Model file for the job. Use its own axes, mm. Coordinates: 2 decimals unless noted, no trailing zeros. Write each loop counter-clockwise with the first axis right and the second up, starting at its lowest first coordinate (ties: lowest second). Pieces come first, ordered by that corner, then holes. Notation, with made-up numbers: (70, 70) -> (92, 70) arc R27 cw to (92, 93) -> close; hole circle Ø3 at (-31, 69). An arc over 180 degrees is marked (long way). Answer as a JSON object with one key per item and string values. Group by question number.
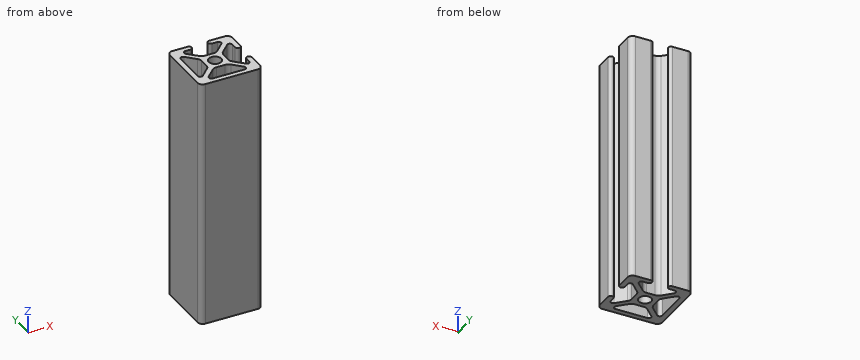
Autodesk Inventor part; units mm, degrees
ref_plane "YZ Plane" through (0, 0, 0) normal (1, 0, 0) x (0, 1, 0)
ref_plane "XZ Plane" through (0, 0, 0) normal (0, 1, 0) x (-1, 0, 0)
ref_plane "XY Plane" through (0, 0, 0) normal (0, 0, 1) x (1, 0, 0)
sketch "Sketch1" plane through (0, 0, 0) normal (0, 0, 1) x (1, 0, 0)
  arc A0 (-10.36, -6.4282) -> (-8.6498, -7.1366) centre (-9.3582, -6.4282) ccw
  line L0 (-10.36, 6.4282) -> (-10.36, -6.4282)
  arc A1 (-8.6498, 7.1366) -> (-10.36, 6.4282) centre (-9.3582, 6.4282) ccw
  line L1 (-5.1567, 3.6435) -> (-8.6498, 7.1366)
  arc A2 (-4.38, 1.7684) -> (-5.1567, 3.6435) centre (-7.0317, 1.7684) ccw
  line L2 (-4.38, -1.7684) -> (-4.38, 1.7684)
  arc A3 (-5.1567, -3.6435) -> (-4.38, -1.7684) centre (-7.0317, -1.7684) ccw
  line L3 (-8.6498, -7.1366) -> (-5.1567, -3.6435)
  arc A4 (-1.7684, -4.38) -> (-3.6435, -5.1567) centre (-1.7684, -7.0317) ccw
  line L4 (1.7684, -4.38) -> (-1.7684, -4.38)
  arc A5 (3.6435, -5.1567) -> (1.7684, -4.38) centre (1.7684, -7.0317) ccw
  line L5 (7.1366, -8.6498) -> (3.6435, -5.1567)
  arc A6 (6.4282, -10.36) -> (7.1366, -8.6498) centre (6.4282, -9.3582) ccw
  line L6 (-6.4282, -10.36) -> (6.4282, -10.36)
  arc A7 (-7.1366, -8.6498) -> (-6.4282, -10.36) centre (-6.4282, -9.3582) ccw
  line L7 (-3.6435, -5.1567) -> (-7.1366, -8.6498)
  circle A8 centre (0, 0) radius 2.5
  arc A9 (-4.32, 10.36) -> (-4.32, 12.5) centre (-4.32, 11.43) ccw
  line L8 (-4.32, 12.5) -> (-10.5183, 12.5)
  arc A10 (-10.5183, 12.5) -> (-12.5, 10.5183) centre (-10.5183, 10.5183) ccw
  line L9 (-12.5, 10.5183) -> (-12.5, -10.5183)
  arc A11 (-12.5, -10.5183) -> (-10.5183, -12.5) centre (-10.5183, -10.5183) ccw
  line L10 (-10.5183, -12.5) -> (10.5183, -12.5)
  arc A12 (10.5183, -12.5) -> (12.5, -10.5183) centre (10.5183, -10.5183) ccw
  line L11 (12.5, -10.5183) -> (12.5, -4.32)
  arc A13 (12.5, -4.32) -> (10.36, -4.32) centre (11.43, -4.32) ccw
  line L12 (10.36, -4.32) -> (10.36, -6.4282)
  arc A14 (8.6498, -7.1366) -> (10.36, -6.4282) centre (9.3582, -6.4282) ccw
  line L13 (8.6498, -7.1366) -> (5.1567, -3.6435)
  arc A15 (4.38, -1.7684) -> (5.1567, -3.6435) centre (7.0317, -1.7684) ccw
  line L14 (4.38, -1.7684) -> (4.38, 1.7684)
  arc A16 (5.1567, 3.6435) -> (4.38, 1.7684) centre (7.0317, 1.7684) ccw
  line L15 (5.1567, 3.6435) -> (8.6498, 7.1366)
  arc A17 (10.36, 6.4282) -> (8.6498, 7.1366) centre (9.3582, 6.4282) ccw
  line L16 (10.36, 6.4282) -> (10.36, 4.32)
  arc A18 (10.36, 4.32) -> (12.5, 4.32) centre (11.43, 4.32) ccw
  line L17 (12.5, 4.32) -> (12.5, 10.5183)
  arc A19 (12.5, 10.5183) -> (10.5183, 12.5) centre (10.5183, 10.5183) ccw
  line L18 (10.5183, 12.5) -> (4.32, 12.5)
  arc A20 (4.32, 12.5) -> (4.32, 10.36) centre (4.32, 11.43) ccw
  line L19 (4.32, 10.36) -> (6.4282, 10.36)
  arc A21 (7.1366, 8.6498) -> (6.4282, 10.36) centre (6.4282, 9.3582) ccw
  line L20 (7.1366, 8.6498) -> (3.6435, 5.1567)
  arc A22 (1.7684, 4.38) -> (3.6435, 5.1567) centre (1.7684, 7.0317) ccw
  line L21 (1.7684, 4.38) -> (-1.7684, 4.38)
  arc A23 (-3.6435, 5.1567) -> (-1.7684, 4.38) centre (-1.7684, 7.0317) ccw
  line L22 (-3.6435, 5.1567) -> (-7.1366, 8.6498)
  arc A24 (-6.4282, 10.36) -> (-7.1366, 8.6498) centre (-6.4282, 9.3582) ccw
  line L23 (-6.4282, 10.36) -> (-4.32, 10.36)
extrude "Extrusion1" add sketch "Sketch1" against normal blind 100
properties part number "25-2502-BLACK-FB"
(1) Cut at A-A on x = 0. List the corners of the cut face in (y, z), plus the area to 3 significant figures.
(2) Cut at D-D on z = -33.5. Give the number of separate pieces and of enclosed holes in the cut face, plus the area to 3 significant figures.
(3) Cut at B-B on y = 11.43. List the corners of the cut face in (x, z).
(4) Wall check: probe 1 along Y at (x, z) = (0, -28); probe 2 along Y at (x, z) = (6.5, -90.5); probe 3 along X at (y, z) = (-6, -46.5). Give the ranges that are in metal, low to high.
(5) Pin check, flat tips, straight feed: pin 1 (3 mm diameter, centred on x = -0.5, y = -1, fed in from +Z); pin 2 (1.1 mm diameter, centred on y = 0.5, z = -69, fed in from +X); pin 3 (4 mm diameter, centred on x = 0.5, z = -35.5, fed in from +Y); pin 4 (3 mm diameter, centred on x = -2, z = -80.5, fed in from +Y). Stop position of each tip, or through.
Results found:
{
 "1": {"outline": "(-12.5, -100) -> (-10.36, -100) -> (-10.36, 0) -> (-12.5, 0) -> close; (-4.38, -100) -> (-2.5, -100) -> (-2.5, 0) -> (-4.38, 0) -> close; (2.5, -100) -> (4.38, -100) -> (4.38, 0) -> (2.5, 0) -> close", "area": "590 mm²"},
 "2": {"separate pieces": "1", "enclosed holes": "3", "area": "303 mm²"},
 "3": {"outline": "(-12.28, -100) -> (-3.25, -100) -> (-3.25, 0) -> (-12.28, 0) -> close; (3.25, -100) -> (12.28, -100) -> (12.28, 0) -> (3.25, 0) -> close"},
 "4": {"probe 1": "y = -12.5 to -10.36, -4.38 to -2.5, 2.5 to 4.38", "probe 2": "y = -12.5 to -10.36, -8.01 to -4.99, 4.99 to 8.01, 10.36 to 12.5", "probe 3": "x = -12.5 to -10.36, -7.51 to -4.49, 4.49 to 7.51, 10.36 to 12.5"},
 "5": {"pin 1": "stops at z = 0", "pin 2": "stops at x = 4.38", "pin 3": "stops at y = 4.48", "pin 4": "stops at y = 12.12"}
}
